Part model, mm, in its own coordinate system. Face numbers are marked on the shaded views. A direction names the side the tool comes from. Coordinates: 2 decimals unless noted, no trailing zeros. Loops run counter-clockwise (first coordinate to the right, second up) from the corner with the lowest first, then second, coordinate; pieces in that order, holes last. Notation, with made-up numbers: M 64,-37 L 74,-37 A26 cw 74,-1 Z; hole C 2,-9 d8. An arc over 180 degrees is marked long. Answer as CSV lines item,"result". Start each with the question number.
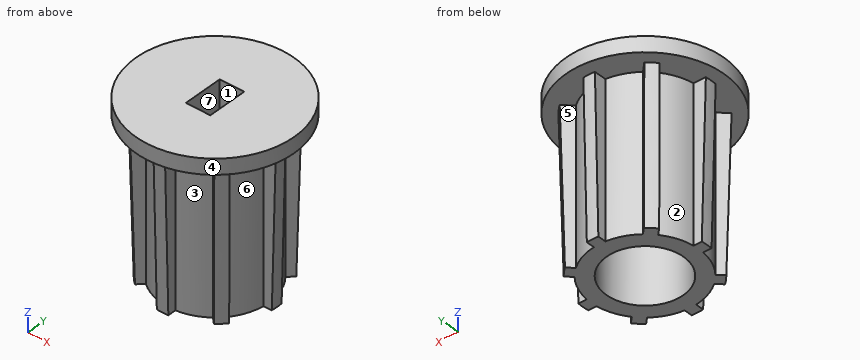
from build123d import *

# Parameters (mm, degrees)
SKETCH_1_R           = 20.6
EXTRUDE_1_DEPTH      = 4
EXTRUDE_2_DEPTH      = 1
EXTRUDE_2_DEPTH_BACK = 40
SKETCH_2_R           = 14
SKETCH_2_R_2         = 10
EXTRUDE_3_DEPTH      = 40
SKETCH_9_R           = 14
EXTRUDE_4_DEPTH      = 14
SKETCH_10_W          = 6.4
SKETCH_10_H          = 10.4
CUT_EXTRUDE_1_DEPTH  = 12
SCALE_1_SCALE        = 0.5


with BuildPart() as part:
    # Sketch 1 → Extrude 1 (new body)
    with BuildSketch(Plane.XY):
        Circle(SKETCH_1_R)
    extrude(amount=EXTRUDE_1_DEPTH)



with BuildPart() as body_2:
    # Sketch 2 → Extrude 2 (new, two sides: drawn at the far end of the back side and taken through both)
    with BuildSketch(Plane.XY.offset(-EXTRUDE_2_DEPTH_BACK)):
        Circle(SKETCH_2_R)
        Circle(SKETCH_2_R_2, mode=Mode.SUBTRACT)
    extrude(amount=EXTRUDE_2_DEPTH + EXTRUDE_2_DEPTH_BACK)


with BuildPart() as part_1:
    add(part.part)

    add(body_2.part)  # Extrude 3 merges body 2
    # Sketch 3 → Extrude 3 (add)
    with BuildSketch(Plane(origin=(0, 0, 0), x_dir=(-1, 0, 0), z_dir=(0, 0, -1))):
        with BuildLine():
            ThreePointArc((-8.753841642, -10.925669613), (-9.881821028, -9.917137347), (-10.894370922, -8.792763059))
            Line((-10.894370922, -8.792763059), (-13.198589674, -11.028926993))
            ThreePointArc((-13.198589674, -11.028926993), (-12.161693133, -12.162780115), (-11.027747345, -13.199575315))
            Line((-11.027747345, -13.199575315), (-8.753841642, -10.925669613))
        make_face()
        with BuildLine():
            ThreePointArc((1.5, -13.919410907), (0, -14), (-1.5, -13.919410907))
            Line((-1.5, -13.919410907), (-1.5, -17.134468186))
            ThreePointArc((-1.5, -17.134468186), (0, -17.2), (1.5, -17.134468186))
            Line((1.5, -17.134468186), (1.5, -13.919410907))
        make_face()
        with BuildLine():
            ThreePointArc((10.894370922, -8.792763059), (9.881821028, -9.917137347), (8.753841642, -10.925669613))
            Line((8.753841642, -10.925669613), (11.027747345, -13.199575315))
            ThreePointArc((11.027747345, -13.199575315), (12.161693133, -12.162780115), (13.198589674, -11.028926993))
            Line((13.198589674, -11.028926993), (10.894370922, -8.792763059))
        make_face()
        with BuildLine():
            Line((17.134468186, 1.5), (13.919410907, 1.5))
            ThreePointArc((13.919410907, 1.5), (13.979838209, 0.751081654), (14, 0))
            ThreePointArc((14, 0), (13.979838209, -0.751081654), (13.919410907, -1.5))
            Line((13.919410907, -1.5), (17.134468186, -1.5))
            ThreePointArc((17.134468186, -1.5), (17.2, 0), (17.134468186, 1.5))
        make_face()
        with BuildLine():
            Line((11.027747345, 13.199575315), (8.753841642, 10.925669613))
            ThreePointArc((8.753841642, 10.925669613), (9.881821028, 9.917137347), (10.894370922, 8.792763059))
            Line((10.894370922, 8.792763059), (13.198589674, 11.028926993))
            ThreePointArc((13.198589674, 11.028926993), (12.161693133, 12.162780115), (11.027747345, 13.199575315))
        make_face()
        with BuildLine():
            Line((-1.5, 17.134468186), (-1.5, 13.919410907))
            ThreePointArc((-1.5, 13.919410907), (0, 14), (1.5, 13.919410907))
            Line((1.5, 13.919410907), (1.5, 17.134468186))
            ThreePointArc((1.5, 17.134468186), (0, 17.2), (-1.5, 17.134468186))
        make_face()
        with BuildLine():
            Line((-13.198589674, 11.028926993), (-10.894370922, 8.792763059))
            ThreePointArc((-10.894370922, 8.792763059), (-9.881821028, 9.917137347), (-8.753841642, 10.925669613))
            Line((-8.753841642, 10.925669613), (-11.027747345, 13.199575315))
            ThreePointArc((-11.027747345, 13.199575315), (-12.161693133, 12.162780115), (-13.198589674, 11.028926993))
        make_face()
        with BuildLine():
            Line((-13.919410907, 1.5), (-17.134468186, 1.5))
            ThreePointArc((-17.134468186, 1.5), (-17.2, 0), (-17.134468186, -1.5))
            Line((-17.134468186, -1.5), (-13.919410907, -1.5))
            ThreePointArc((-13.919410907, -1.5), (-14, 0), (-13.919410907, 1.5))
        make_face()
    extrude(amount=EXTRUDE_3_DEPTH)

    # Sketch 8 → Cut-Revolve 2 (revolve, cut)
    with BuildSketch(Plane(origin=(0, 0, 0), x_dir=(0, 0, -1), z_dir=(1, 0, 0))):
        Polygon((40, 16.152563137), (0, 17.2), (40, 17.2), align=None)
    revolve(axis=Axis((0, 0, 0), (0, 0, -1)), mode=Mode.SUBTRACT)

    # Sketch 9 → Extrude 4 (add)
    with BuildSketch(Plane(origin=(0, 0, 0), x_dir=(-1, 0, 0), z_dir=(0, 0, -1))):
        Circle(SKETCH_9_R)
    extrude(amount=EXTRUDE_4_DEPTH)

    # Sketch 10 → Cut-Extrude 1 (cut)
    with BuildSketch(Plane.XY.offset(4)):
        Rectangle(SKETCH_10_W, SKETCH_10_H)
    extrude(amount=-CUT_EXTRUDE_1_DEPTH, mode=Mode.SUBTRACT)


with BuildPart() as part_2:
    # Scale 1: scaled about (0, 0, -13.067917949)
    add(part_1.part.scale(SCALE_1_SCALE).moved(Location((0, 0, -6.533958974))))


solid = part_2.part
Q1. Tool access for the marked faces 5, 6 and 7: list every direction of +Z, -Z, +X, -X, +Y, -Y with a clear straight run to the whole face (end or side of a thin tool).
Q2. Slice it at B-B, the plane x = 0. Write the cut outline in (y, z), and give its area (3 significant figures).
Q3. Two-plate mould, pull along Y, no slides. Class the marked faces 1, 2, 3 and 4: +Y half, -Y half, draft (parallel to the pull), parting line (faces both ways), or undercut.
Q4. Slice it at C-C, the plane y = -1.25. Write the cut outline in (x, z).
Q5. Flat gauge pins, fed straight in: P1, Ø0.8, axis at y = 8, z = -14, coming from the +X side; P2, Ø1.5, axis at x = -3, z = -18, coming from the -Y side; P3, Ø1, axis at x = 0, y = -0.5, coming from the +Z side. Where does each tip first touch, or does it go through?
Q6. Wall check: L1, parallel to X at y = 5.75, z = -22.5; L2, parallel to Z at x = 6.75, y = 3; L3, parallel to X at y = -4.5, z = -15.5. Give the ranges that are in metal, low to high.
Solved:
1,face 5,"-Z, +Y"
1,face 6,"-Z, +X"
1,face 7,"+Z"
2,outline,"M -10.3,-6.53 L -8.6,-6.53 L -8.08,-26.53 L -5,-26.53 L -5,-13.53 L 5,-13.53 L 5,-26.53 L 8.08,-26.53 L 8.6,-6.53 L 10.3,-6.53 L 10.3,-4.53 L 2.6,-4.53 L 2.6,-10.53 L -2.6,-10.53 L -2.6,-4.53 L -10.3,-4.53 Z"
2,area,"214 mm2"
3,face 1,"undercut"
3,face 2,"undercut"
3,face 3,"-Y half"
3,face 4,"parting line"
4,outline,"M -10.22,-6.53 L -6.89,-6.53 L -6.89,-26.53 L -4.84,-26.53 L -4.84,-13.53 L 4.84,-13.53 L 4.84,-26.53 L 6.89,-26.53 L 6.89,-6.53 L 10.22,-6.53 L 10.22,-4.53 L 1.6,-4.53 L 1.6,-10.53 L -1.6,-10.53 L -1.6,-4.53 L -10.22,-4.53 Z"
5,P1,"stops at x = 0.75"
5,P2,"stops at y = -6.63"
5,P3,"stops at z = -10.53"
6,L1,"x = -5.82 to -4.66, -3.99 to 3.99, 4.66 to 5.82"
6,L2,"z = -6.53 to -4.53"
6,L3,"x = -5.55 to -2.18, 2.18 to 5.55"
